Geometry: final body of the model. Coordinates: model frame, mm. A direction names the side the tool comes from. Coordinates: 2 decimals unless noted, no trailing zeros. Order: outer loops, then holes, each group sorted by start corner. A loop starts at its lowest first (then second) coordinate and runs counter-clockwise, first axis right, second up. Notation, with made-up numbers: (8.5, -30.75) -> (38.5, -30.75) arc R9 ccw to (38.5, -17.75) -> close; hole circle Ø2 at (19, -17). An arc over 180 degrees is marked (long way). Use one line per item in the form item = value.
```python
from build123d import *

# Parameters (mm, degrees)
EXTRUDE_THIN1_DEPTH = 381
FILLET1_R           = 1.27


with BuildPart() as part:
    # Sketch1 → Extrude-Thin1 (new body)
    with BuildSketch(Plane.XY):
        with BuildLine():
            Line((0, 34.13125), (0, 38.1))
            Line((0, 38.1), (-20.6375, 38.1))
            Line((-20.6375, 38.1), (-20.6375, 26.9875))
            Line((-20.6375, 26.9875), (-16.66875, 26.9875))
            Line((-16.66875, 26.9875), (-16.66875, 24.60625))
            ThreePointArc((-16.66875, 24.60625), (-20.637199415, 19.108011605), (-16.556782099, 13.692348143))
            ThreePointArc((-16.556782099, 13.692348143), (-9.182459335, 8.539010459), (-6.35, 0))
            Line((-6.35, 0), (0, 0))
            Line((0, 0), (0, 4.365625))
            Line((0, 4.365625), (-1.27, 4.365625))
            Line((-1.27, 4.365625), (-1.27, 1.27))
            Line((-1.27, 1.27), (-5.131923382, 1.27))
            ThreePointArc((-5.131923382, 1.27), (-8.5544739, 9.799810535), (-16.194051619, 14.909445755))
            ThreePointArc((-16.194051619, 14.909445755), (-19.348945082, 19.572203738), (-15.39875, 23.58351569))
            Line((-15.39875, 23.58351569), (-15.39875, 28.2575))
            Line((-15.39875, 28.2575), (-19.3675, 28.2575))
            Line((-19.3675, 28.2575), (-19.3675, 36.83))
            Line((-19.3675, 36.83), (-1.27, 36.83))
            Line((-1.27, 36.83), (-1.27, 34.13125))
            Line((-1.27, 34.13125), (0, 34.13125))
        make_face()
    extrude(amount=-EXTRUDE_THIN1_DEPTH)

    # Fillet1
    fillet1_edges = [part.edges().sort_by_distance(p)[0] for p in [
        (0, 0, -190.5),
        (-6.35, 0, -190.5),
        (-20.6375, 26.9875, -190.5),
        (-20.6375, 38.1, -190.5),
        (0, 38.1, -190.5),
        (-15.39875, 28.2575, -190.5),
        (-15.39875, 23.58351569, -190.5),
    ]]
    fillet(fillet1_edges, radius=FILLET1_R)


solid = part.part
```
1) Contact query for flat-ended pins moving along their axis: P1, Ø1, axis at x = -0.5, z = -238, coming from the +Y side; P2, Ø2, axis at x = -18, z = -173.5, coming from the -Y side; P3, Ø12, axis at y = 14, z = -104, coming from the +X side. Output: stop coordinate, or through.
Results found:
P1 = 38.07
P2 = 13.84
P3 = -7.29
2) Material intervals for probe 1 along Y at (x, z) = (-3.75, -284); probe 2 along X at (y, z) = (36.5, -269.5); probe 3 along X at (y, z) = (18.5, -192), sorted ascending. Write a range as from..to.
Results found:
probe_1 = 0..1.27, 36.83..38.1
probe_2 = -20.64..-19.37, -1.27..0
probe_3 = -20.6..-19.32
3) Section A-A, the plane x = -12. Output: boundary loops of the cut face in (y, z), and give its area (3 significant figures).
Results found:
outline = (11.38, -381) -> (12.94, -381) -> (12.94, 0) -> (11.38, 0) -> close; (36.83, -381) -> (38.1, -381) -> (38.1, 0) -> (36.83, 0) -> close
area = 1,080 mm2
4) Pull-direction query (X, two-part tool) for faces 3 (the cylindrical face through (-8.473, 9.698, -187.833)), 4 (the flat face through (-10, 38.1, -188)), 5 (the cylindrical face through (-9.617, 9.093, -187.833)); classes: released by +X, released by -X, zero draft, split by the parting line, or undercut.
Results found:
face_3 = undercut
face_4 = zero draft
face_5 = released by -X
5) Section B-B, the plane z = -195. Output: boundary loops of the cut face in (x, y) (1 decimal), and give its area (3 significant figures).
Results found:
outline = (-20.6, 28.3) arc R1.3 ccw to (-19.4, 27) -> (-16.7, 27) -> (-16.7, 24.6) arc R5.7 ccw to (-16.6, 13.7) arc R14.3 cw to (-6.4, 1.2) arc R1.3 ccw to (-5.1, 0) -> (-1.3, 0) arc R1.3 ccw to (0, 1.3) -> (0, 4.4) -> (-1.3, 4.4) -> (-1.3, 1.3) -> (-5.1, 1.3) arc R15.6 ccw to (-16.2, 14.9) arc R4.4 cw to (-16.3, 23.4) arc R1.3 ccw to (-15.4, 24.6) -> (-15.4, 27) arc R1.3 ccw to (-16.7, 28.3) -> (-19.4, 28.3) -> (-19.4, 36.8) -> (-1.3, 36.8) -> (-1.3, 34.1) -> (0, 34.1) -> (0, 36.8) arc R1.3 ccw to (-1.3, 38.1) -> (-19.4, 38.1) arc R1.3 ccw to (-20.6, 36.8) -> close
area = 100 mm2
6) Section C-C, the plane y = 10. Output: boundary loops of the cut face in (x, z), and give its area (3 significant figures).
Results found:
outline = (-10.43, -381) -> (-8.72, -381) -> (-8.72, 0) -> (-10.43, 0) -> close
area = 653 mm2
7) Access query for faces 1 (the flat face through (-19.368, 32, -188)), 2 (the flat face through (-20.638, 33, -188)). Directions: +Z, -Z, +X, -X, +Y, -Y. A direction counts if a zero-diameter tool reaches every point of the face in a straight line with its end or side. Return the directions, or none.
Results found:
face_1 = +Z, -Z
face_2 = +Z, -Z, -X, +Y, -Y
